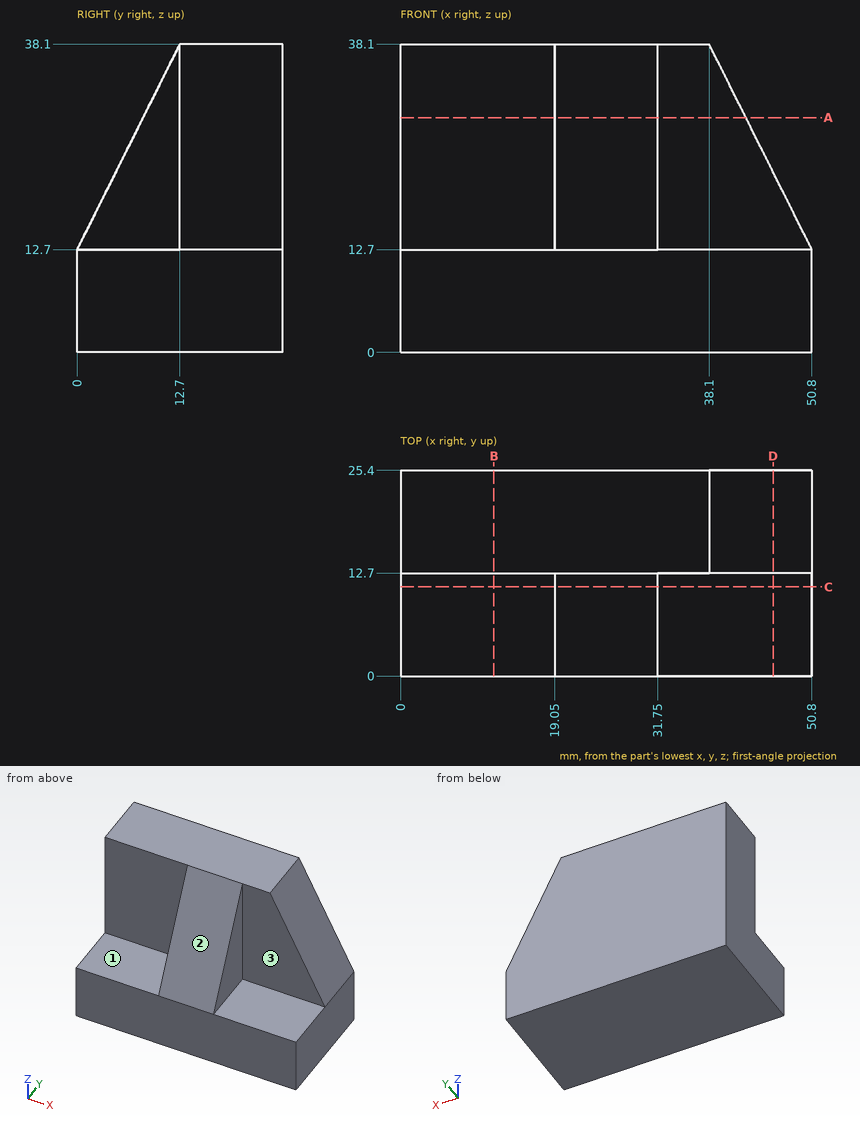
Answer from the drawing. Dimensions are ordinates in mm from the lowest x, y and z of the part. A direction names the side the tool comes from. Give positions to 0.01 mm unless a question says otherwise; leave off trailing zeros. Order: outer loops, then holes, each group sorted by start corner. A loop starts at its lowest first (then second) coordinate and runs counter-clockwise, first axis right, second up.
(1) Find section A-A (z = 29). Give the vertices of the cut face in (x, y), plus the area to 3 significant figures.
(2) Find section D-D (x = 46). Give the vertices of the cut face in (y, z).
(3) Straight lines are drawn through the part: L1, parallel to Z at x = 7, y = 2.25; L2, parallel to Y at x = 42, z = 17.5; L3, parallel to X at y = 2.25, z = 17. For each, find the intervals that lie inside material, in ascending order.
(4) Find section B-B (x = 11.5). Give the vertices of the cut face in (y, z), plus the area to 3 significant figures.
(5) Given pin 1 (10 mm diameter, centred on y = 7, z = 29.5, fed in from -X); pin 2 (21 mm diameter, centred on x = 8, z = 30, fed in from -Y); pin 3 (14 mm diameter, centred on y = 8, z = 27, fed in from +X), each flat-ended and moving along its own axis, determine where each tip first touches the part or whether it passes through.
(6) Find section C-C (y = 11). Give the vertices of the cut face in (x, z), plus the area to 3 significant figures.
(7) For the marked faces 1, 2 and 3, determine the directions among +Z, -Z, +X, -X, +Y, -Y from which every point of the face is accessible in a straight line to the end or side of a thin tool.
Result sheet:
1. outline: (0, 12.7) - (19.05, 12.7) - (19.05, 8.15) - (31.75, 8.15) - (31.75, 12.7) - (42.65, 12.7) - (42.65, 25.4) - (0, 25.4) - close
1. area: 599 mm2
2. outline: (0, 0) - (25.4, 0) - (25.4, 22.3) - (12.7, 22.3) - (12.7, 12.7) - (0, 12.7) - close
3. L1: z = 0 to 12.7
3. L2: y = 12.7 to 25.4
3. L3: x = 19.05 to 31.75
4. outline: (0, 0) - (25.4, 0) - (25.4, 38.1) - (12.7, 38.1) - (12.7, 12.7) - (0, 12.7) - close
4. area: 645 mm2
5. pin 1: stops at x = 19.05
5. pin 2: stops at y = 12.7
5. pin 3: stops at x = 46.24
6. outline: (0, 0) - (50.8, 0) - (50.8, 12.7) - (31.75, 12.7) - (31.75, 34.7) - (19.05, 34.7) - (19.05, 12.7) - (0, 12.7) - close
6. area: 925 mm2
7. face 1: +Z, -X, -Y
7. face 2: +Z, +X, -X, -Y
7. face 3: +Z, +X, -Y
